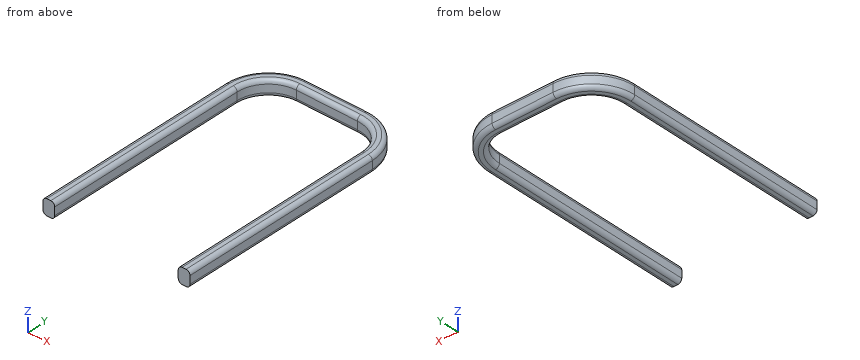
from build123d import *

# Parameters (mm, degrees)
F1_W = 0.75
F1_H = 1
F3_R = 0.25


with BuildPart() as f2:
    # F2: sweep along a path in F0
    with BuildLine(Plane.XY) as f2_path:
        Line((-3.95, 0), (-3.95, 13))
        ThreePointArc((-3.95, 13), (-3.3642135624, 14.4142135624), (-1.95, 15))
        Line((-1.95, 15), (1.95, 15))
        ThreePointArc((1.95, 15), (3.3642135624, 14.4142135624), (3.95, 13))
        Line((3.95, 13), (3.95, 0))
    # F1 (on Front) → F2 (sweep)
    with BuildSketch(Plane.XZ):
        with Locations((-4.325, 0.5)):
            Rectangle(F1_W, F1_H)
    sweep(path=f2_path.line)

    # F3
    f3_edges = [f2.edges().sort_by_distance(p)[0] for p in [
        (-4.7, 6.5, 1),
        (-3.95, 6.5, 1),
        (3.95, 6.5, 0),
        (4.7, 6.5, 0),
    ]]
    fillet(f3_edges, radius=F3_R)


solid = f2.part
Check sheet for the modelled part. Datum: model origin and axes. Units: mm. Round coordinates to 2 decimals unless told otherwise and drop trailing zeros. Order: outer loops, then holes, each group sorted by start corner. A loop starts at its lowest first (then second) coordinate and runs counter-clockwise, first axis right, second up.
(1) Cross-section at C-C, the plane z = 0.4. Enter the section's corners in (x, y), and give its area (3 significant figures).
(2) Cross-section at B-B, the plane x = -0.25. Enter the section's corners in (y, z).
(3) Scan lines: probe 1 along X at (y, z) = (12.5, 0.25); probe 2 along Y at (x, z) = (-1.5, 0.7). Record each from-to range of solid material in increasing order.
(4) Cross-section at A-A, the plane y = 6.5. Enter the section's corners in (x, z), and give its area (3 significant figures).
Check sheet entries:
1. outline: (-4.7, 0) - (-3.95, 0) - (-3.95, 13) arc R2 cw to (-1.95, 15) - (1.95, 15) arc R2 cw to (3.95, 13) - (3.95, 0) - (4.7, 0) - (4.7, 13) arc R2.75 ccw to (1.95, 15.75) - (-1.95, 15.75) arc R2.75 ccw to (-4.7, 13) - close
1. area: 28.0 mm2
2. outline: (15, 0.25) arc R0.25 ccw to (15.25, 0) - (15.5, 0) arc R0.25 ccw to (15.75, 0.25) - (15.75, 0.75) arc R0.25 ccw to (15.5, 1) - (15.25, 1) arc R0.25 ccw to (15, 0.75) - close
3. probe 1: x = -4.7 to -3.95, 3.95 to 4.7
3. probe 2: y = 15 to 15.75
4. outline: (-4.7, 0.25) arc R0.25 ccw to (-4.45, 0) - (-4.2, 0) arc R0.25 ccw to (-3.95, 0.25) - (-3.95, 0.75) arc R0.25 ccw to (-4.2, 1) - (-4.45, 1) arc R0.25 ccw to (-4.7, 0.75) - close; (3.95, 0.25) arc R0.25 ccw to (4.2, 0) - (4.45, 0) arc R0.25 ccw to (4.7, 0.25) - (4.7, 0.75) arc R0.25 ccw to (4.45, 1) - (4.2, 1) arc R0.25 ccw to (3.95, 0.75) - close
4. area: 1.39 mm2
